Study the drawing (mm; zero at the part's minimum x, y, z) and answer. Coordinates: 2 decimals unless noted, no trailing zeros. Loops run counter-clockwise (first coordinate to the right, second up) from the corner with the lowest first, then second, coordinate; pieces in that order, holes last. Notation, with made-up numbers: (2, 17.5) -> (45, 17.5) arc R7 ccw to (45, 27.5) -> close; hole circle Ø11 at (-3.75, 9). An arc over 180 degrees is marked (long way). Answer as a JSON object with one key per item and string values. Group by question number.
Q1. The part is cut by section C-C on y = 9.25. Write down the section's boundary in (x, z), and give its area (3 significant figures).
Q2. The part is cut by section A-A on x = 3.85. Write down the section's boundary in (y, z).
Q3. This flat-tipped pin is pushed along its axis until it touches: P1, Ø2.5, axis at y = 11, z = 51, coming from the +X side. Where does it stop, or does it pass through?
Q4. Straight lines are drawn through the part: line 1 along Z through (x, y) = (3.1, 10); line 2 along Z through (x, y) = (3.9, 13); line 3 along Y through (x, z) = (2.65, 50.5). For each, find the intervals that lie inside material, in ascending order. Write a range as [from, to].
Q5. The part is cut by section B-B on z = 47. Write down the section's boundary in (x, y), and give its area (3 significant figures).
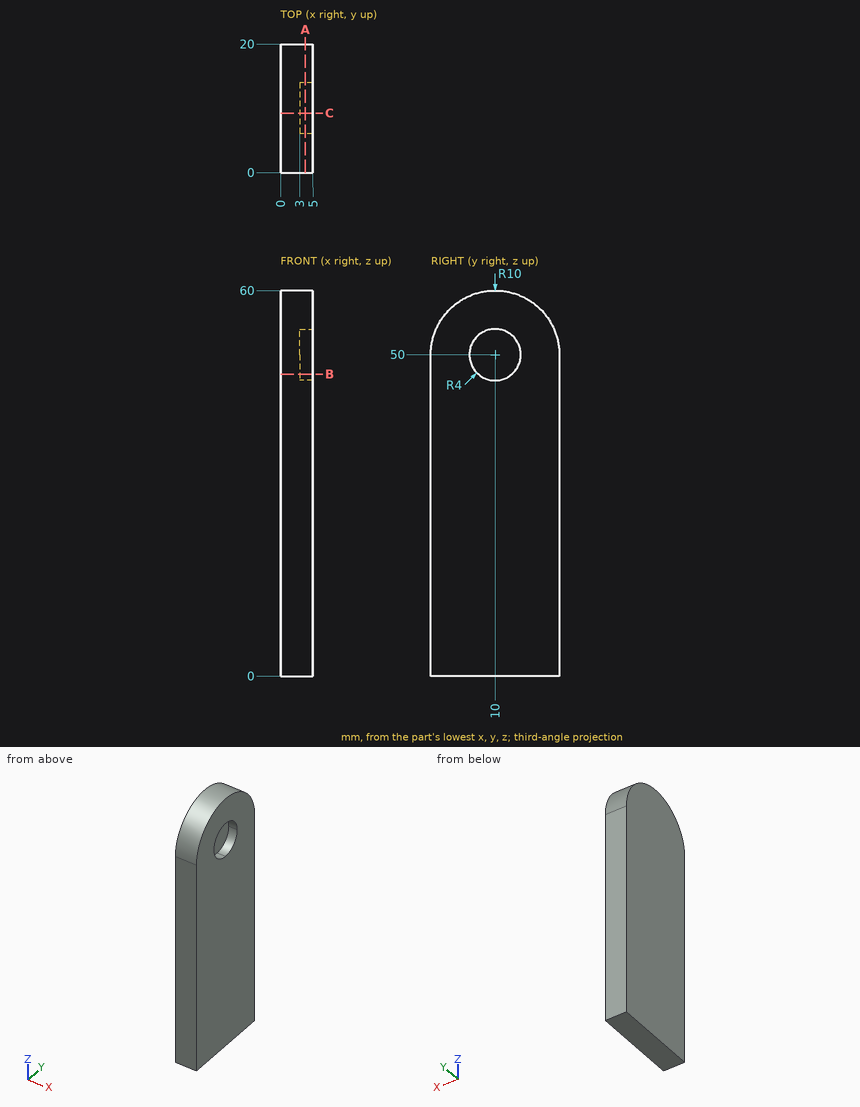
Final values:
{
 "1": {"outline": "(0, 0) -> (5, 0) -> (5, 46.07) -> (3, 46.07) -> (3, 53.93) -> (5, 53.93) -> (5, 59.97) -> (0, 59.97) -> close", "area": "284 mm2"},
 "2": {"outline": "(0, 0) -> (20, 0) -> (20, 50) arc R10 ccw to (0, 50) -> close; hole circle Ø8 at (10, 50)"},
 "3": {"P1": "stops at x = 3"},
 "4": {"line 1": "z = [0, 46], [54, 60]", "line 2": "z = [0, 47.35], [52.65, 59.54]", "line 3": "y = [0.01, 19.99]"},
 "5": {"outline": "(0, 0) -> (5, 0) -> (5, 7.35) -> (3, 7.35) -> (3, 12.65) -> (5, 12.65) -> (5, 20) -> (0, 20) -> close", "area": "89.4 mm2"}
}
